Verification items for the finished model (mm, model axes). A direction names the side the tool comes from. Round coordinates to 2 decimals unless told otherwise and drop trailing zeros. Write each loop counter-clockwise with the first axis right and the second up, starting at its lowest first coordinate (ties: lowest second). Pieces come first, ordered by that corner, then holes. Notation, with made-up numbers: (6.25, 31.5) -> (45.25, 31.5) arc R22 cw to (45.25, 58.5) -> close; hole circle Ø2 at (38.25, 42). An arc over 180 degrees is marked (long way). Answer as a JSON object with one key per item and string values. Group by question number.
(1) Gauge pin test, flat ends, axial feed: pin 1 Ø1 at (x, y) = (-10.5, 5) entering from -Z; pin 2 Ø8 at (x, y) = (2, 37) entering from -Z; pin 3 Ø8 at (y, z) = (7, -21.5) entering from -X; pin 4 Ø5.5 at (x, z) = (0, 0) entering from -Y. Record the tip position at first contact, or that the pin passes through.
(2) Scan lines: L1, parallel to Z at x = 0, y = 3 (3 decimals); L2, parallel to Y at x = 10, z = -7; L3, parallel to Z at x = 0, y = 20. Record each from-to range of solid material in increasing order. Write a range as from..to.
(3) Sectioned sample at B-B on z = 0. Record the cut outline in (x, y) (3 decimals), and give its area (3 significant figures).
(4) Sectioned sample at D-D on x = 8.5. Record the cut outline in (y, z) (3 decimals).
(5) Draft check along X on faces 6 (the face through (-12.69, 43.65, -0.51)), 7 (the face through (-4.544, 6.512, -0.151)), 8 (the face through (-12, 17.018, 5)). Enter one of: released by +X, released by -X, zero draft, split by the parting line, or undercut.
(6) Sectioned sample at C-C on y = 16. Record the cut outline in (x, z) (3 decimals).
(7) Set-up check for faces 1 (the face through (-12.2, 41.783, 0.1)), 2 (the face through (0, 0, 6)), 3 (the face through (-6.346, 28.983, -0.233)), 4 (the face through (12, 12, -3.175)), 5 (the face through (-3, 44.323, 6)): record each of +Z, -Z, +X, -X, +Y, -Y from which the full face is reachable in a straight line by a thin tool's end or side.
(8) Sectioned sample at A-A on x = 0. Record the cut outline in (y, z) (3 decimals).
```python
from build123d import *

# Parameters (mm, degrees)
SKETCH1_R           = 27.305
SKETCH1_R_2         = 4.5466
BOSS_EXTRUDE1_DEPTH = 57.658
SKETCH2_R           = 6.35
CUT_EXTRUDE1_DEPTH  = 44.45
SKETCH3_OUTSIDE_W   = 75.886
SKETCH3_OUTSIDE_H   = 75.886
SKETCH3_OUTSIDE_R   = 12.7
CUT_EXTRUDE2_DEPTH  = 44.45
SKETCH10_W          = 30.679481275
SKETCH10_H          = 6.35
CUT_EXTRUDE7_DEPTH  = 6.35
SKETCH13_OUTSIDE_W  = 75.886
SKETCH13_OUTSIDE_H  = 75.886
SKETCH13_OUTSIDE_R  = 11.938
CUT_EXTRUDE9_DEPTH  = 1.1684
SKETCH16_R          = 46.08237905
CUT_EXTRUDE11_DEPTH = 14.335
SKETCH18_R          = 16.51
SKETCH18_R_2        = 12.7
BOSS_EXTRUDE4_DEPTH = 3.81
SKETCH19_OUTSIDE_W  = 74.42
SKETCH19_OUTSIDE_H  = 74.42
SKETCH19_OUTSIDE_R  = 16.51
CUT_EXTRUDE12_DEPTH = 1.27
SKETCH10_2_W        = 30.679481275
SKETCH10_2_H        = 6.35
CUT_EXTRUDE13_DEPTH = 45.323


with BuildPart() as part:
    # Sketch1 → Boss-Extrude1 (new body)
    with BuildSketch(Plane(origin=(0, 0, 0), x_dir=(1, 0, 0), z_dir=(0, 1, 0))):
        Circle(SKETCH1_R)
        Circle(SKETCH1_R_2, mode=Mode.SUBTRACT)
    extrude(amount=BOSS_EXTRUDE1_DEPTH)

    # Sketch2 → Cut-Extrude1 (cut)
    with BuildSketch(Plane(origin=(0, 57.658, 0), x_dir=(1, 0, 0), z_dir=(0, 1, 0))):
        Circle(SKETCH2_R)
    extrude(amount=-CUT_EXTRUDE1_DEPTH, mode=Mode.SUBTRACT)

    # Sketch3 outside → Cut-Extrude2 (cut)
    with BuildSketch(Plane(origin=(0, 57.658, 0), x_dir=(1, 0, 0), z_dir=(0, 1, 0))):
        Rectangle(SKETCH3_OUTSIDE_W, SKETCH3_OUTSIDE_H)
        Circle(SKETCH3_OUTSIDE_R, mode=Mode.SUBTRACT)
    extrude(amount=-CUT_EXTRUDE2_DEPTH, mode=Mode.SUBTRACT)

    # Sketch10 → Cut-Extrude7 (cut)
    with BuildSketch(Plane.XZ):
        with Locations((17.839550223, 0)):
            Rectangle(SKETCH10_W, SKETCH10_H)
    extrude(amount=-CUT_EXTRUDE7_DEPTH, mode=Mode.SUBTRACT)

    # Sketch13 outside → Cut-Extrude9 (cut)
    with BuildSketch(Plane(origin=(0, 41.783, 0), x_dir=(-1, 0, 0), z_dir=(0, 1, 0))):
        Rectangle(SKETCH13_OUTSIDE_W, SKETCH13_OUTSIDE_H)
        Circle(SKETCH13_OUTSIDE_R, mode=Mode.SUBTRACT)
    extrude(amount=CUT_EXTRUDE9_DEPTH, mode=Mode.SUBTRACT)

    # Sketch16 → Cut-Extrude11 (cut, through all)
    with BuildSketch(Plane(origin=(0, 44.323, 0), x_dir=(-1, 0, 0), z_dir=(0, 1, 0))):
        Circle(SKETCH16_R)
    extrude(amount=CUT_EXTRUDE11_DEPTH, mode=Mode.SUBTRACT)

    # Sketch18 → Boss-Extrude4 (add)
    with BuildSketch(Plane(origin=(0, 13.208, 0), x_dir=(1, 0, 0), z_dir=(0, 1, 0))):
        Circle(SKETCH18_R)
        Circle(SKETCH18_R_2, mode=Mode.SUBTRACT)
    extrude(amount=BOSS_EXTRUDE4_DEPTH)

    # Sketch19 outside → Cut-Extrude12 (cut)
    with BuildSketch(Plane(origin=(0, 13.208, 0), x_dir=(1, 0, 0), z_dir=(0, 1, 0))):
        Rectangle(SKETCH19_OUTSIDE_W, SKETCH19_OUTSIDE_H)
        Circle(SKETCH19_OUTSIDE_R, mode=Mode.SUBTRACT)
    extrude(amount=-CUT_EXTRUDE12_DEPTH, mode=Mode.SUBTRACT)

    # Sketch10_2 → Cut-Extrude13 (cut, through all)
    with BuildSketch(Plane.XZ):
        with Locations((17.839550223, 0)):
            Rectangle(SKETCH10_2_W, SKETCH10_2_H)
    extrude(amount=-CUT_EXTRUDE13_DEPTH, mode=Mode.SUBTRACT)


solid = part.part
```
Computed values:
{
 "1": {"pin 1": "z = -25.41", "pin 2": "z = -12.7", "pin 3": "x = -20.96", "pin 4": "through"},
 "2": {"L1": "-27.305..-4.547, 4.547..27.305", "L2": "0..41.78, 42.95..44.32", "L3": "-12.7..-6.35, 6.35..12.7"},
 "3": {"outline": "(-27.305, 0) -> (-4.547, 0) -> (-4.547, 13.208) -> (-6.35, 13.208) -> (-6.35, 44.323) -> (-12.7, 44.323) -> (-12.7, 42.951) -> (-11.938, 42.951) -> (-11.938, 41.783) -> (-12.7, 41.783) -> (-12.7, 17.018) -> (-16.51, 17.018) -> (-16.51, 11.938) -> (-27.305, 11.938) -> close", "area": "498 mm2"},
 "4": {"outline": "(0, -25.948) -> (11.938, -25.948) -> (11.938, -14.154) -> (17.018, -14.154) -> (17.018, -9.436) -> (41.783, -9.436) -> (41.783, -8.382) -> (42.951, -8.382) -> (42.951, -9.436) -> (44.323, -9.436) -> (44.323, -3.175) -> (0, -3.175) -> close; (0, 3.175) -> (44.323, 3.175) -> (44.323, 9.436) -> (42.951, 9.436) -> (42.951, 8.382) -> (41.783, 8.382) -> (41.783, 9.436) -> (17.018, 9.436) -> (17.018, 14.154) -> (11.938, 14.154) -> (11.938, 25.948) -> (0, 25.948) -> close"},
 "5": {"face 6": "split by the parting line", "face 7": "undercut", "face 8": "zero draft"},
 "6": {"outline": "(5.499, -3.175) arc R6.35 cw (long way) to (5.499, 3.175) -> (16.202, 3.175) arc R16.51 ccw (long way) to (16.202, -3.175) -> close"},
 "7": {"face 1": "none", "face 2": "+Z, -Z, +X, -X, -Y", "face 3": "+Y", "face 4": "+X, +Y, -Y", "face 5": "+Z, -Z, +X, -X, +Y"},
 "8": {"outline": "(0, -27.305) -> (11.938, -27.305) -> (11.938, -16.51) -> (17.018, -16.51) -> (17.018, -12.7) -> (41.783, -12.7) -> (41.783, -11.938) -> (42.951, -11.938) -> (42.951, -12.7) -> (44.323, -12.7) -> (44.323, -6.35) -> (13.208, -6.35) -> (13.208, -4.547) -> (0, -4.547) -> close; (0, 4.547) -> (13.208, 4.547) -> (13.208, 6.35) -> (44.323, 6.35) -> (44.323, 12.7) -> (42.951, 12.7) -> (42.951, 11.938) -> (41.783, 11.938) -> (41.783, 12.7) -> (17.018, 12.7) -> (17.018, 16.51) -> (11.938, 16.51) -> (11.938, 27.305) -> (0, 27.305) -> close"}
}
